Work out the finished part from the listing and answer in its coordinate system (mm). Give positions to 0.01 mm unless a question says otherwise; leave off trailing zeros. Loops run counter-clockwise (first coordinate to the right, second up) from the corner with the lowest first, then second, coordinate; pieces in that order, holes last.
```python
from build123d import *

# Parameters (mm, degrees)
F0_R     = 0.4
F1_DEPTH = 0.49


with BuildPart() as f1:
    # F0 (on Front) → F1 (new body)
    with BuildSketch(Plane.XZ):
        Polygon((0.5, 3), (-1, 3), (-1, -1), (3.4, -1), (3.4, -1.5), (6.7, -1.5), (7.2, -1), (7.9, -1.7), (8.6, -1), (16.2, -1), (16.2, -0.5), (18.2, -0.5), (18.2, 1), (8.6, 1), (7.9, 1.7), (7.2, 1), (6.7, 1.5), (5.25, 1.5), (5.25, 7.5), (4.9, 7.5), (4.9, 10), (3.4, 10), (3.4, 4.5), (3.8, 4.5), (3.8, 1), (0.5, 1), align=None)
        Circle(F0_R, mode=Mode.SUBTRACT)
        with Locations((13.2, 0)):
            Circle(F0_R, mode=Mode.SUBTRACT)
    extrude(amount=F1_DEPTH)


solid = f1.part
```
Q1. Section B-B on z = 2.75 is taken. Give the vertices of the cut face in (x, y).
Q2. Section C-C on x = 0 is taken. Give the vertices of the cut face in (y, z), plus the area to 3 significant figures.
Q3. Consider line 1 along X through (y, z) = (-0.2, 2); line 2 along Z through (x, y) = (0, -0.3); line 3 along Z through (x, y) = (13.2, -0.3). Determine where each line is inside the solid, lowest interval first.
Q4. Section A-A on y = -0.1 is taken. Give the vertices of the cut face in (x, z), plus the area to 3 significant figures.
Q5. Section D-D on z = 0 is taken. Give the vertices of the cut face in (x, y), plus the area to 3 significant figures.
Check result:
1. outline: (-1, -0.49) - (0.5, -0.49) - (0.5, 0) - (-1, 0) - close; (3.8, -0.49) - (5.25, -0.49) - (5.25, 0) - (3.8, 0) - close
2. outline: (-0.49, -1) - (0, -1) - (0, -0.4) - (-0.49, -0.4) - close; (-0.49, 0.4) - (0, 0.4) - (0, 3) - (-0.49, 3) - close
2. area: 1.57 mm2
3. line 1: x = -1 to 0.5, 3.8 to 5.25
3. line 2: z = -1 to -0.4, 0.4 to 3
3. line 3: z = -1 to -0.4, 0.4 to 1
4. outline: (-1, -1) - (3.4, -1) - (3.4, -1.5) - (6.7, -1.5) - (7.2, -1) - (7.9, -1.7) - (8.6, -1) - (16.2, -1) - (16.2, -0.5) - (18.2, -0.5) - (18.2, 1) - (8.6, 1) - (7.9, 1.7) - (7.2, 1) - (6.7, 1.5) - (5.25, 1.5) - (5.25, 7.5) - (4.9, 7.5) - (4.9, 10) - (3.4, 10) - (3.4, 4.5) - (3.8, 4.5) - (3.8, 1) - (0.5, 1) - (0.5, 3) - (-1, 3) - close; hole circle Ø0.8 at (0, 0); hole circle Ø0.8 at (13.2, 0)
4. area: 57.4 mm2
5. outline: (-1, -0.49) - (-0.4, -0.49) - (-0.4, 0) - (-1, 0) - close; (0.4, -0.49) - (12.8, -0.49) - (12.8, 0) - (0.4, 0) - close; (13.6, -0.49) - (18.2, -0.49) - (18.2, 0) - (13.6, 0) - close
5. area: 8.62 mm2
